Design review of the part shown in the three views and the two pictorial views. Dimensions are in mm from the part's minimum x, y and z. Coordinates: 2 decimals unless noted, no trailing zeros. Write each loop counter-clockwise with the first axis right and the second up, starting at its lowest first coordinate (ties: lowest second). Pieces come first, ordered by that corner, then holes.
Q1. For L1, parallel to Z at x = 75, y = 2.6; L2, parallel to Z at x = 34, y = 3.6; L3, parallel to Z at x = 112, y = 4.4 (1 decimal), list the stretches that pass through material, from the lowest coordinate up.
Q2. Take a section at B-B, the plane z = 38. Write out the cut boundary in (x, y), plus the area to 3 significant figures.
Q3. Take a section at C-C, the plane y = 2.25. State how many separate pieces and enclosed holes the cut face has, plus the area to 3 significant figures.
Q4. For pin 1 Ø3 at (y, z) = (1.5, 39.5) entering from -X; pin 2 Ø7.5 at (x, z) = (36.11, 36.11) entering from +Y; pin 3 Ø1 at (x, y) = (62.5, 4) entering from -Z, all flat-tipped, find the tip position at first contact; note any pin that passes through.
Q5. Take a section at D-D, the plane z = 64.5. Write out the cut boundary in (x, y) (1 decimal).
Q6. Take a section at A-A, the plane x = 75. Write out the cut boundary in (y, z), plus the area to 3 significant figures.
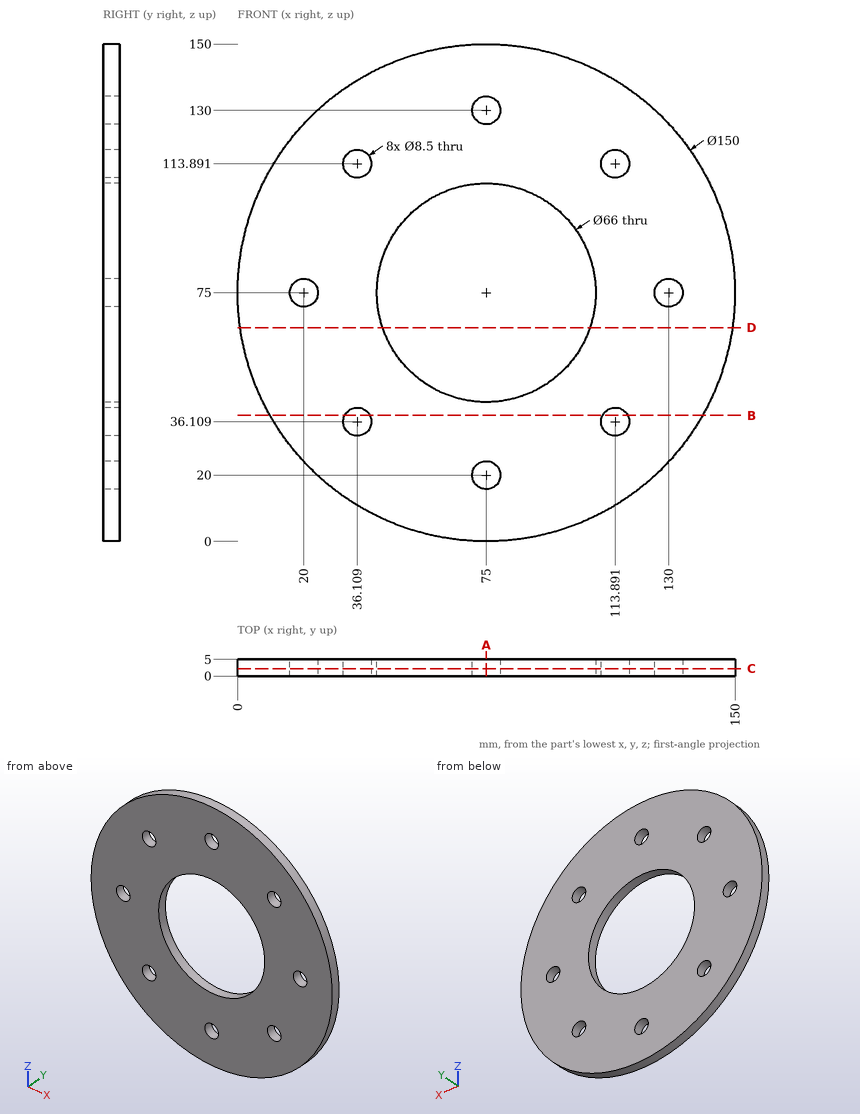
Responses:
1. L1: z = 0 to 15.75, 24.25 to 42, 108 to 125.75, 134.25 to 150
1. L2: z = 12.2 to 32.42, 39.8 to 110.2, 117.58 to 137.8
1. L3: z = 9.8 to 32.3, 39.9 to 110.1, 117.7 to 140.2
2. outline: (9.76, 0) - (32.3, 0) - (32.3, 5) - (9.76, 5) - close; (39.92, 0) - (110.08, 0) - (110.08, 5) - (39.92, 5) - close; (117.7, 0) - (140.24, 0) - (140.24, 5) - (117.7, 5) - close
2. area: 576 mm2
3. separate pieces: 1
3. enclosed holes: 9
3. area: 13,800 mm2
4. pin 1: stops at x = 8.15
4. pin 2: passes through
4. pin 3: stops at z = 0.97
5. outline: (0.7, 0) - (43.7, 0) - (43.7, 5) - (0.7, 5) - close; (106.3, 0) - (149.3, 0) - (149.3, 5) - (106.3, 5) - close
6. outline: (0, 0) - (5, 0) - (5, 15.75) - (0, 15.75) - close; (0, 24.25) - (5, 24.25) - (5, 42) - (0, 42) - close; (0, 108) - (5, 108) - (5, 125.75) - (0, 125.75) - close; (0, 134.25) - (5, 134.25) - (5, 150) - (0, 150) - close
6. area: 335 mm2
